Can you work these out from the drawing? Everything is in mm from the part's minimum corner. Coordinates: 2 decimals unless noted, no trailing zeros. Order: outer loops, then holes, each group sorted by start corner. A loop starts at its lowest first (then second) coordinate and runs counter-clockwise, first axis right, second up. Notation, with made-up numbers: (-4, -22.75) - (21, -22.75) arc R27 ccw to (21, 4.25) - close; hole circle Ø7 at (71, 89). An arc over 180 degrees is marked (long way). Answer as CSV lines item,"result". Start each with the question number.
Item 1: Imagine slicing it at B-B on x = 16.25. List the corners of the cut face in (y, z) for me (3 decimals), and give its area (3 significant figures).
Item 2: I need wall thicknesses on line 1 (Z direction, x = 15.25, y = 1.95) (3 decimals); line 2 (X direction, y = 2.2, z = 7); line 3 (Z direction, x = 23, y = 1). Which ranges of each line are inside material? Lowest first, please.
Item 3: Imagine slicing it at A-A on y = 1.1. List the corners of the cut face in (x, z) for me (3 decimals).
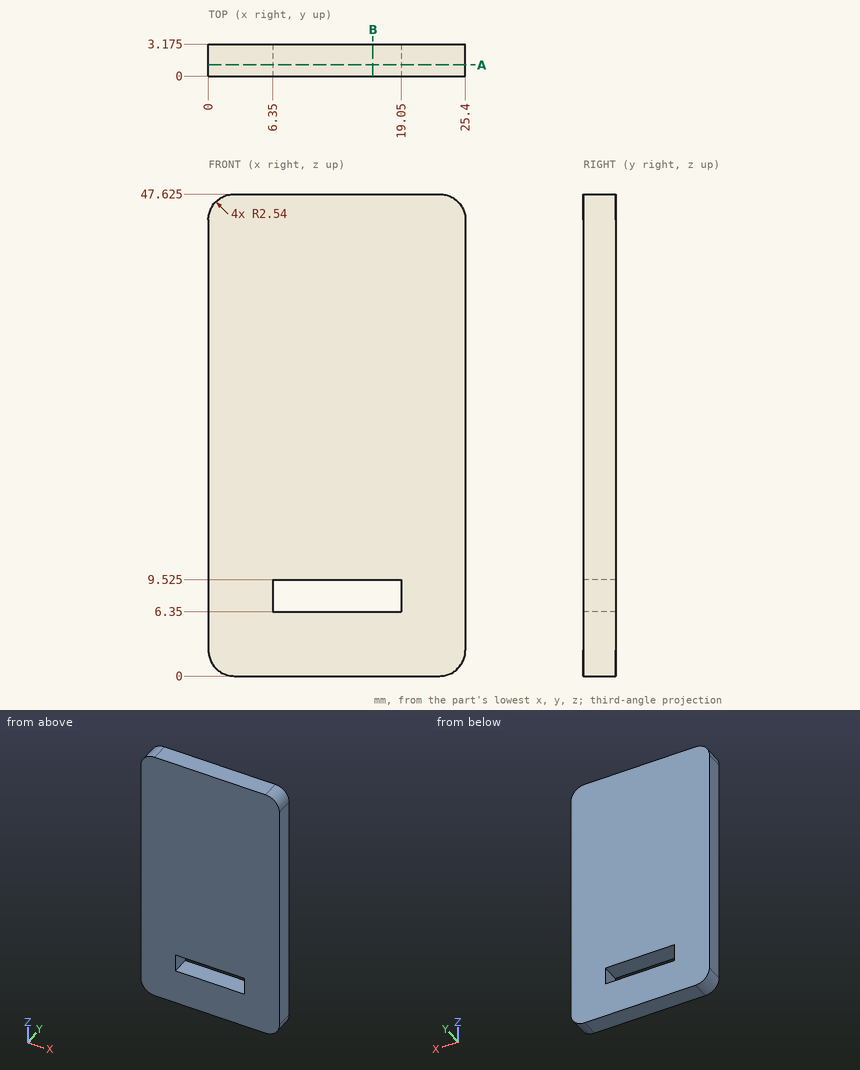
Responses:
1,outline,"(0, 0) - (3.175, 0) - (3.175, 6.35) - (0, 6.35) - close; (0, 9.525) - (3.175, 9.525) - (3.175, 47.625) - (0, 47.625) - close"
1,area,"141 mm^2"
2,line 1,"z = 0 to 6.35, 9.525 to 47.625"
2,line 2,"x = 0 to 6.35, 19.05 to 25.4"
2,line 3,"z = 0 to 47.62"
3,outline,"(0, 2.54) arc R2.54 ccw to (2.54, 0) - (22.86, 0) arc R2.54 ccw to (25.4, 2.54) - (25.4, 45.085) arc R2.54 ccw to (22.86, 47.625) - (2.54, 47.625) arc R2.54 ccw to (0, 45.085) - close; hole (6.35, 6.35) - (19.05, 6.35) - (19.05, 9.525) - (6.35, 9.525) - close"
